Here's how the part is built. I have some questions about the finished solid (model axes, mm). A direction names the side the tool comes from. Give positions to 0.01 mm unless a question says otherwise; leave off trailing zeros. Write each loop counter-clockwise with the first axis right and the second up, starting at its lowest first coordinate (ties: lowest second). Pieces come first, ordered by that corner, then holes. Notation, with made-up numbers: (-6, 49.5) - (45, 49.5) arc R32 ccw to (45, 78.5) - close; hole circle Ø6 at (-37.5, -0.75). An arc over 180 degrees is marked (long way). Write each question's results on one line, items separated by ' | '. Start each with the question number.
Item 1: Which directions (+Z, -Z, +X, -X, +Y, -Y) give clear straight access to the entire face, cutting with the end or side of a thin tool? Please do faces 1 (the flat face through (1, 4.9, 1)), 2 (the flat face through (0, 0, 1.15)).
Item 2: Suppose I cut it at B-B on x = 7.5. List the corners of the cut face in (y, z) for me, then the cut area to 3 significant figures.
Item 3: Suppose I cut it at A-A on y = 2. List the corners of the cut face in (x, z) for me.
Item 4: Please list where this line runs through material, in increasing order: line 1 along Z through (x, y) = (-9.5, -1).
```python
from build123d import *

# Parameters (mm, degrees)
SKETCH_1_W      = 30
SKETCH_1_H      = 11.5
SKETCH_1_W_2    = 25.9
SKETCH_1_H_2    = 8.8
SKETCH_1_W_3    = 22.384
SKETCH_1_H_3    = 5.584
EXTRUDE_2_DEPTH = 1.2
SKETCH_1_6_W    = 22.384
SKETCH_1_6_H    = 5.584
EXTRUDE_4_DEPTH = 1.15


with BuildPart() as part:
    # Sketch 1 → Extrude 2 (new body)
    with BuildSketch(Plane.XY):
        with Locations((1.7, -0.85)):
            Rectangle(SKETCH_1_W, SKETCH_1_H)
        Rectangle(SKETCH_1_W_2, SKETCH_1_H_2, mode=Mode.SUBTRACT)
        Rectangle(SKETCH_1_W_2, SKETCH_1_H_2)
        Rectangle(SKETCH_1_W_3, SKETCH_1_H_3, mode=Mode.SUBTRACT)
    extrude(amount=EXTRUDE_2_DEPTH)

    # Sketch 1_6 → Extrude 4 (add)
    with BuildSketch(Plane.XY):
        Rectangle(SKETCH_1_6_W, SKETCH_1_6_H)
    extrude(amount=EXTRUDE_4_DEPTH)


solid = part.part
```
Checked values:
1) face 1: +Z, -Z, +X, -X, +Y | face 2: +Z
2) outline: (-6.6, 0) - (4.9, 0) - (4.9, 1.2) - (2.79, 1.2) - (2.79, 1.15) - (-2.79, 1.15) - (-2.79, 1.2) - (-6.6, 1.2) - close | area: 13.5 mm^2
3) outline: (-13.3, 0) - (16.7, 0) - (16.7, 1.2) - (11.19, 1.2) - (11.19, 1.15) - (-11.19, 1.15) - (-11.19, 1.2) - (-13.3, 1.2) - close
4) line 1: z = 0 to 1.15
